Can you work these out from the model? Positions are in its coordinate system, mm. A direction names the side the tool comes from. Give positions to 0.01 mm unless a question says otherwise; leave off trailing zeros. Loops run counter-clockwise (first coordinate to the right, second up) from the corner with the lowest first, then second, coordinate; pieces in that order, holes last. Notation, with made-up numbers: (11, 36) -> (18, 36) arc R20 ccw to (18, 41) -> close; hole circle Ø5 at (16, 39). An arc over 180 degrees is marked (long way). Return JSON: item names as keys, results as strings. Group by question number.
Q1. I need wall thicknesses on line 1 along X through (y, z) = (0, 0.75); line 2 along Y through (x, z) = (0, -0.25); line 3 along Y through (x, z) = (0, -1.5). Which ranges of each line are inside material? Lowest first, please. Write a range as [from, to].
Q2. Will these pins go through, and if not, where does the flat tip stop? pin 1 (3 mm diameter, centred on x = -53.5, y = -0.5, fed in from +Z); pin 2 (2 mm diameter, centred on x = -16, y = 5.5, fed in from +Z); pin 3 (2 mm diameter, centred on x = -6, y = 2.5, fed in from -Z); pin 4 (6 mm diameter, centred on x = -44, z = 3, fed in from -Y).
Q3. Which directions (+Z, -Z, +X, -X, +Y, -Y) give clear straight access to the entire face, cutting with the end or side of a thin tool? Please do faces 1 (the flat face through (-58, 0, 0)), 2 (the flat face through (-43, 0, 6)).
Q4. Suppose I cut it at B-B, the plane z = 0. Please give me the cut outline in (x, y).
Q5. Suppose I cut it at D-D, the plane x = 0. Please give me the cut outline in (y, z), and give its area (3 significant figures).
Q6. Suppose I cut it at A-A, the plane y = 0. Please give me the cut outline in (x, z), and give its area (3 significant figures).
Q7. Suppose I cut it at C-C, the plane x = -17.5. Please give me the cut outline in (y, z).
Q8. Thinking about a two-plate mould opening in X: for faces 3 (the flat face through (5, 0, 0)), 4 (the cylindrical face through (-2.91, 2.67, -0.1)), 5 (the flat face through (-51, 0, 5)), which applies, pulls with the +X half, pulls with the -X half, needs draft (parallel to the pull), parting line crosses it, or undercut?
```python
from build123d import *

# Parameters (mm, degrees)
ESQUISSE1_W                  = 63
ESQUISSE1_H                  = 7
CHANFREIN1_SIZE              = 1
ENL_V_MAT_EXTRU_2_DEPTH      = 10
ENL_V_MAT_EXTRU_2_DEPTH_BACK = 10
ESQUISSE2_R                  = 3.95
ESQUISSE3_W                  = 3
ESQUISSE3_H                  = 13
ENL_V_MAT_EXTRU_3_DEPTH      = 15


with BuildPart() as part:
    # Esquisse1 → Base-Révolution (revolve)
    with BuildSketch(Plane.XY, mode=Mode.PRIVATE) as base_r_volution_sk:
        with Locations((-26.5, 3.5)):
            Rectangle(ESQUISSE1_W, ESQUISSE1_H)
    revolve(base_r_volution_sk.sketch.rotate(Axis((9, 0, 0), (-1, 0, 0)), 314.415308597), axis=Axis((9, 0, 0), (-1, 0, 0)))

    # Chanfrein1
    chanfrein1_edges = [part.edges().sort_by_distance(p)[0] for p in [
        (5, -4.898979486, -5),
    ]]
    chamfer(chanfrein1_edges, length=CHANFREIN1_SIZE)

    # Esquisse2 → Enlèv. mat.-Extru.2 (cut, two sides: drawn at the far end of the back side and taken through both)
    with BuildSketch(Plane.XY.offset(-ENL_V_MAT_EXTRU_2_DEPTH_BACK)):
        Circle(ESQUISSE2_R)
    extrude(amount=ENL_V_MAT_EXTRU_2_DEPTH + ENL_V_MAT_EXTRU_2_DEPTH_BACK, mode=Mode.SUBTRACT)

    # Esquisse3 → Enlèv. mat.-Extru.3 (cut)
    with BuildSketch(Plane.ZY.offset(58)):
        with Locations((6.5, 0.5)):
            Rectangle(ESQUISSE3_W, ESQUISSE3_H)
    extrude(amount=-ENL_V_MAT_EXTRU_3_DEPTH, mode=Mode.SUBTRACT)


solid = part.part
```
Ans:
{
 "1": {"line 1": "x = [-58, -3.95], [3.95, 5]", "line 2": "y = [-7, -3.95], [3.95, 7]", "line 3": "y = [-6.84, -3.95], [3.95, 6.84]"},
 "2": {"pin 1": "stops at z = 5", "pin 2": "stops at z = 5.36", "pin 3": "stops at z = -6.84", "pin 4": "stops at y = -7"},
 "3": {"face 1": "+Z, -Z, -X, +Y, -Y", "face 2": "+Z, -X, +Y, -Y"},
 "4": {"outline": "(-58, -7) -> (4, -7) -> (5, -6) -> (5, 6) -> (4, 7) -> (-58, 7) -> close; hole circle Ø7.9 at (0, 0)"},
 "5": {"outline": "(-3.95, -5.78) -> (-3.95, 5.78) arc R7 ccw to start; (3.95, -5.78) arc R7 ccw to (3.95, 5.78) -> close", "area": "49.5 mm^2"},
 "6": {"outline": "(-58, -7) -> (-3.95, -7) -> (-3.95, 7) -> (-43, 7) -> (-43, 5) -> (-58, 5) -> close; (3.95, -7) -> (4, -7) -> (5, -6) -> (5, 6) -> (4, 7) -> (3.95, 7) -> close", "area": "740 mm^2"},
 "7": {"outline": "circle Ø14 at (0, 0)"},
 "8": {"face 3": "pulls with the +X half", "face 4": "undercut", "face 5": "needs draft"}
}
